Part model, mm, in its own coordinate system. Face numbers are marked on the shaded views. A direction names the side the tool comes from. Round coordinates to 2 decimals unless told otherwise and drop trailing zeros. Loops run counter-clockwise (first coordinate to the right, second up) from the corner with the lowest first, then second, coordinate; pieces in that order, holes last. Notation, with made-up numbers: M 86,52.5 L 91,52.5 A17 ccw 91,60.5 Z; hole C 73,58 d5. An arc over 180 degrees is marked long. Answer as CSV lines item,"result". Start each with the question number.
Item 1: Mould opens along X. For the marked faces 1, 2 and 3 say: pulls with the +X half, pulls with the -X half, needs draft (parallel to the pull), parting line crosses it, or undercut.
Item 2: Band-saw the part on B-B (z = -19.5). Give the cut face in (x, y), and give its area (3 significant figures).
Item 3: Drop flat-ended pins along their axis: pin 1 Ø8 at (x, z) = (23, -18.5) entering from -Y; pin 2 Ø4 at (x, y) = (35, 30) entering from +Z; pin 3 Ø1.5 at (x, z) = (10.5, -24) entering from +Y; pin 4 Ø4 at (y, z) = (12, 2) entering from -X. Give the stop position or say it passes through.
Item 4: Wall check: line 1 (X direction, y = 24.5, z = -3.5); line 2 (Y direction, x = 22.5, z = -2); line 3 (Z direction, x = 17.5, y = -5). Give the ranges that are in metal, low to high.
Item 5: Which spindle directions (+Z, -Z, +X, -X, +Y, -Y) get a long thin tool onto all of the face, cutting with end or side? Do the marked faces 4, 5 and 6. Say none if no direction does.
Item 6: Band-saw the part on C-C (y = -29.5). Give the cut face in (x, z), and give its area (3 significant figures).
Item 7: Band-saw the part on A-A (x = 14). Give the cut face in (y, z), and give its area (3 significant figures).
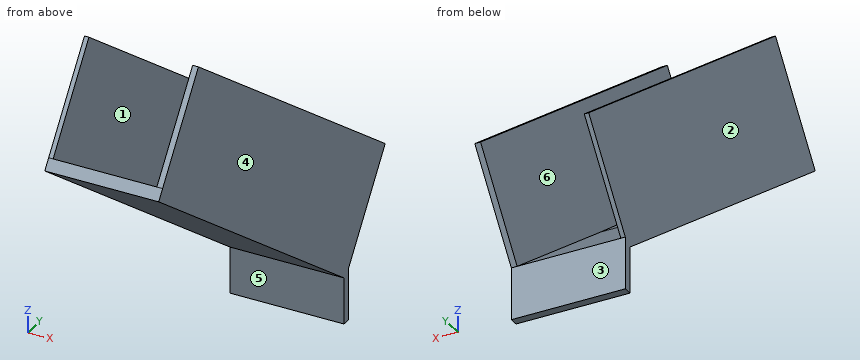
```python
from build123d import *

# Parameters (mm, degrees)
BOSS_EXTRUDE1_DEPTH = 40
SKETCH4_W           = 1.560342198
SKETCH4_H           = 149.198591979
BOSS_EXTRUDE2_DEPTH = 40
SKETCH6_W           = 2.027300843
SKETCH6_H           = 149.198591979
BOSS_EXTRUDE3_DEPTH = 40


with BuildPart() as part:
    # Sketch3 → Boss-Extrude1 (new body)
    with BuildSketch(Plane(origin=(0, 0, 0), x_dir=(0, 0, -1), z_dir=(1, 0, 0))):
        Polygon((0, 0), (39.348289754, 53.871692839), (57.75585878, 53.871692839), (57.75585878, 50.831910798), (41.374811114, 50.831910798), (-45.883583059, -68.633444315), (-49.329231032, -66.116717112), align=None)
    extrude(amount=BOSS_EXTRUDE1_DEPTH)

    # Sketch4 → Boss-Extrude2 (add)
    with BuildSketch(Plane(origin=(0, 0, 0), x_dir=(1, 0, 0), z_dir=(0, 0.5898261654750604, 0.8075302437190738))):
        with Locations((0.780171099, -7.887623879)):
            Rectangle(SKETCH4_W, SKETCH4_H)
    extrude(amount=BOSS_EXTRUDE2_DEPTH)

    # Sketch6 → Boss-Extrude3 (add)
    with BuildSketch(Plane(origin=(0, 0, 0), x_dir=(1, 0, 0), z_dir=(0, 0.5898261654750604, 0.8075302437190738))):
        with Locations((38.986349578, -7.887623879)):
            Rectangle(SKETCH6_W, SKETCH6_H)
    extrude(amount=BOSS_EXTRUDE3_DEPTH)


solid = part.part
```
Answer block:
1,face 1,"undercut"
1,face 2,"pulls with the -X half"
1,face 3,"needs draft"
2,outline,"M 0,20.88 L 40,20.88 L 40,68.37 L 37.97,68.37 L 37.97,26.7 L 1.56,26.7 L 1.56,68.37 L 0,68.37 Z"
2,area,"382 mm^2"
3,pin 1,"stops at y = 14.04"
3,pin 2,"stops at z = -20.45"
3,pin 3,"stops at y = 33.89"
3,pin 4,"stops at x = 0"
4,line 1,"x = 0 to 1.56, 37.97 to 40"
4,line 2,"y = -3.08 to 2.74"
4,line 3,"z = -0.59 to 3.73"
5,face 4,"+Z, -Z, +X, +Y, -Y"
5,face 5,"-Z, +X, -X, -Y"
5,face 6,"+Z, +Y"
6,outline,"M 0,17.3 L 40,17.3 L 40,71.08 L 37.97,71.08 L 37.97,22.01 L 1.56,22.01 L 1.56,71.08 L 0,71.08 Z"
6,area,"364 mm^2"
7,outline,"M -68.63,45.88 L 50.83,-41.37 L 50.83,-57.76 L 53.87,-57.76 L 53.87,-39.35 L 0,0 L -66.12,49.33 Z"
7,area,"597 mm^2"
